Geometry check sheet. Reference: the model listing, model coordinates, mm. Round coordinates to 2 decimals unless told otherwise and drop trailing zeros. Loops run counter-clockwise (first coordinate to the right, second up) from the corner with the lowest first, then second, coordinate; pieces in that order, holes last.
```python
from build123d import *

# Parameters (mm, degrees)
F0_R         = 2.5
F1_DEPTH     = 1
F2_T1_DEPTH  = 10
F2_T4_ANGLE  = 180
F2_T10_ANGLE = 180


# Not quite as in the source:
# - a fillet or chamfer that OpenCascade refuses, or shapes differently, is made with other operations: its cross-section is extruded or revolved along the edge and cut away or added


with BuildPart() as f1:
    # F0 (on Top) → F1 (new body)
    with BuildSketch(Plane.XY):
        with BuildLine():
            Line((5, 4), (-5, 4))
            ThreePointArc((-5, 4), (-9, 0), (-5, -4))
            Line((-5, -4), (5, -4))
            ThreePointArc((5, -4), (9, 0), (5, 4))
        make_face()
        with Locations((-5, 0)):
            Circle(F0_R, mode=Mode.SUBTRACT)
        with Locations((5, 0)):
            Circle(F0_R, mode=Mode.SUBTRACT)
    extrude(amount=F1_DEPTH)

    # F2: fillet of radius 1 on 3 edges, made by hand

    # F2_s2 → F2_t1 (cut)
    with BuildSketch(Plane.YZ.offset(-5)):
        with BuildLine():
            ThreePointArc((4, 0), (3.7071067812, 0.7071067812), (3, 1))
            Line((3, 1), (4, 1))
            Line((4, 1), (4, 0))
        make_face()
        with BuildLine():
            ThreePointArc((-4, 0), (-3.7071067812, 0.7071067812), (-3, 1))
            Line((-3, 1), (-4, 1))
            Line((-4, 1), (-4, 0))
        make_face()
    extrude(amount=F2_T1_DEPTH, mode=Mode.SUBTRACT)

    # F2_s3 → F2_t4 (revolve, cut)
    with BuildSketch(Plane.YZ.offset(-5)):
        with BuildLine():
            ThreePointArc((4, 0), (3.7071067812, 0.7071067812), (3, 1))
            Line((3, 1), (4, 1))
            Line((4, 1), (4, 0))
        make_face()
    revolve(axis=Axis((-5, 0, 1), (0, 0, 1)), revolution_arc=F2_T4_ANGLE, mode=Mode.SUBTRACT)

    # F2_s5 → F2_t6 (revolve, cut)
    with BuildSketch(Plane.XZ):
        with BuildLine():
            ThreePointArc((-2.5, 0), (-2.2071067812, 0.7071067812), (-1.5, 1))
            Line((-1.5, 1), (-2.5, 1))
            Line((-2.5, 1), (-2.5, 0))
        make_face()
    revolve(axis=Axis((-5, 0, 1), (0, 0, 1)), mode=Mode.SUBTRACT)

    # F2_s7 → F2_t8 (revolve, cut)
    with BuildSketch(Plane.XZ):
        with BuildLine():
            ThreePointArc((7.5, 0), (7.7928932188, 0.7071067812), (8.5, 1))
            Line((8.5, 1), (7.5, 1))
            Line((7.5, 1), (7.5, 0))
        make_face()
    revolve(axis=Axis((5, 0, 1), (0, 0, 1)), mode=Mode.SUBTRACT)

    # F2_s9 → F2_t10 (revolve, cut)
    with BuildSketch(Plane.YZ.offset(5)):
        with BuildLine():
            ThreePointArc((-4, 0), (-3.7071067812, 0.7071067812), (-3, 1))
            Line((-3, 1), (-4, 1))
            Line((-4, 1), (-4, 0))
        make_face()
    revolve(axis=Axis((5, 0, 1), (0, 0, 1)), revolution_arc=F2_T10_ANGLE, mode=Mode.SUBTRACT)


solid = f1.part
```
1) Scan lines: line 1 along X through (y, z) = (1, 0.65); line 2 along X through (y, z) = (-2, 0.35); line 3 along Y through (x, z) = (5.25, 0.45) (3 decimals). Record each from-to range of solid material in increasing order.
Report:
line 1: x = -8.62 to -7.55, -2.45 to 2.45, 7.55 to 8.62
line 2: x = -8.39 to -6.6, -3.4 to 3.4, 6.6 to 8.39
line 3: y = -3.885 to -2.595, 2.595 to 3.885
2) Sectioned sample at B-B, the plane x = -1.25. Record the cut outline in (y, z), then the cut area to 3 significant figures.
Report:
outline: (-4, 0) - (4, 0) arc R1 ccw to (3, 1) - (-3, 1) arc R1 ccw to start
area: 7.57 mm2
3) Sectioned sample at A-A, the plane z = 0.8. Record the cut outline in (x, y), then the cut area to 3 significant figures.
Report:
outline: (-5, -3.6) - (5, -3.6) arc R3.6 ccw to (5, 3.6) - (-5, 3.6) arc R3.6 ccw to start; hole circle Ø5.8 at (-5, 0); hole circle Ø5.8 at (5, 0)
area: 59.9 mm2
